```python
from build123d import *

# Parameters (mm, degrees)
SKETCH1_W           = 25.5
SKETCH1_H           = 5.5
BOSS_EXTRUDE1_DEPTH = 5


with BuildPart() as part:
    # Sketch1 → Boss-Extrude1 (new body)
    with BuildSketch(Plane.XY):
        Polygon((-100, 151.5), (-100, 146.5), (10, 146.5), (10, 151.5), (30, 151.5), (30, -10), (10, -10), (10, -5), (-100, -5), (-100, -10), (-120, -10), (-120, -5), (-115, -5), (-115, 146.5), (-120, 146.5), (-120, 151.5), align=None)
        with Locations((-58.25, 13.75)):
            Rectangle(SKETCH1_W, SKETCH1_H, mode=Mode.SUBTRACT)
        with Locations((-12.75, 2.75)):
            Rectangle(SKETCH1_W, SKETCH1_H, mode=Mode.SUBTRACT)
        with Locations((-58.25, 2.75)):
            Rectangle(SKETCH1_W, SKETCH1_H, mode=Mode.SUBTRACT)
        with Locations((-12.75, 13.75)):
            Rectangle(SKETCH1_W, SKETCH1_H, mode=Mode.SUBTRACT)
        with Locations((-12.75, 26.25)):
            Rectangle(SKETCH1_W, SKETCH1_H, mode=Mode.SUBTRACT)
        with Locations((-58.25, 26.25)):
            Rectangle(SKETCH1_W, SKETCH1_H, mode=Mode.SUBTRACT)
        with Locations((-58.25, 37.25)):
            Rectangle(SKETCH1_W, SKETCH1_H, mode=Mode.SUBTRACT)
        with Locations((-12.75, 37.25)):
            Rectangle(SKETCH1_W, SKETCH1_H, mode=Mode.SUBTRACT)
        with Locations((-12.75, 49.75)):
            Rectangle(SKETCH1_W, SKETCH1_H, mode=Mode.SUBTRACT)
        with Locations((-58.25, 49.75)):
            Rectangle(SKETCH1_W, SKETCH1_H, mode=Mode.SUBTRACT)
        with Locations((-58.25, 60.75)):
            Rectangle(SKETCH1_W, SKETCH1_H, mode=Mode.SUBTRACT)
        with Locations((-12.75, 60.75)):
            Rectangle(SKETCH1_W, SKETCH1_H, mode=Mode.SUBTRACT)
        with Locations((-12.75, 73.25)):
            Rectangle(SKETCH1_W, SKETCH1_H, mode=Mode.SUBTRACT)
        with Locations((-58.25, 73.25)):
            Rectangle(SKETCH1_W, SKETCH1_H, mode=Mode.SUBTRACT)
        with Locations((-58.25, 84.25)):
            Rectangle(SKETCH1_W, SKETCH1_H, mode=Mode.SUBTRACT)
        with Locations((-12.75, 84.25)):
            Rectangle(SKETCH1_W, SKETCH1_H, mode=Mode.SUBTRACT)
        with Locations((-12.75, 96.75)):
            Rectangle(SKETCH1_W, SKETCH1_H, mode=Mode.SUBTRACT)
        with Locations((-58.25, 96.75)):
            Rectangle(SKETCH1_W, SKETCH1_H, mode=Mode.SUBTRACT)
        with Locations((-58.25, 107.75)):
            Rectangle(SKETCH1_W, SKETCH1_H, mode=Mode.SUBTRACT)
        with Locations((-12.75, 107.75)):
            Rectangle(SKETCH1_W, SKETCH1_H, mode=Mode.SUBTRACT)
        with Locations((-12.75, 120.25)):
            Rectangle(SKETCH1_W, SKETCH1_H, mode=Mode.SUBTRACT)
        with Locations((-58.25, 120.25)):
            Rectangle(SKETCH1_W, SKETCH1_H, mode=Mode.SUBTRACT)
        with Locations((-58.25, 131.25)):
            Rectangle(SKETCH1_W, SKETCH1_H, mode=Mode.SUBTRACT)
        with Locations((-12.75, 131.25)):
            Rectangle(SKETCH1_W, SKETCH1_H, mode=Mode.SUBTRACT)
    extrude(amount=BOSS_EXTRUDE1_DEPTH)


solid = part.part
```
Build history of the part. All positions in model axes, mm. Coordinates: 2 decimals unless noted, no trailing zeros. Order: outer loops, then holes, each group sorted by start corner. A loop starts at its lowest first (then second) coordinate and runs counter-clockwise, first axis right, second up. Notation, with made-up numbers: (87.25, -2) -> (136.25, -2) arc R13 cw to (136.25, 23) -> close; hole circle Ø10 at (-38.75, 54). An arc over 180 degrees is marked (long way). Answer in a Markdown table with one row per item. Add a question column.
Q1. Band-saw the part on D-D, the plane x = -81. List the corners of the cut face in (y, z), then the cut area to 4 significant figures.
Q2. Mould opens along Y. For faces 1 (the face through (-45.5, 108, 2)), 2 (the face through (20, 151.5, 2)), 3 (the face through (10, -8, 2)) say: +Y half, -Y half, draft (parallel to the pull), parting line (faces both ways), or undercut.
Q3. Band-saw the part on A-A, the plane z = 1.7. Give the number of separate pieces and of enclosed holes in the cut face, then the cut area to 3 significant figures.
Q4. Drop flat-ended pins along their axis: pin 1 (2.5 mm diameter, centred on y = 119.5, z = 3, fed in from -X); pin 2 (2.5 mm diameter, centred on x = -6.5, z = 3, fed in from +Y). Give the stop position or say it passes through.
Q5. Wall check: line 1 along X through (y, z) = (95.5, 2.7); line 2 along X through (y, z) = (141, 4.1); line 3 along Y through (x, z) = (-73.5, 1.5). Give the ranges that are in metal, low to high. Write a range as [from, to].
Q6. Band-saw the part on C-C, the plane y = 115.5. List the corners of the cut face in (x, z), then the cut area to 3 significant figures.
Answers follow:
| question | item | result |
|---|---|---|
| 1 | outline | (-5, 0) -> (146.5, 0) -> (146.5, 5) -> (-5, 5) -> close |
| 1 | area | 757.5 mm^2 |
| 2 | face 1 | undercut |
| 2 | face 2 | +Y half |
| 2 | face 3 | draft |
| 3 | separate pieces | 1 |
| 3 | enclosed holes | 24 |
| 3 | area | 19,000 mm^2 |
| 4 | pin 1 | x = -115 |
| 4 | pin 2 | y = 146.5 |
| 5 | line 1 | [-115, -71], [-45.5, -25.5], [0, 30] |
| 5 | line 2 | [-115, 30] |
| 5 | line 3 | [-5, 146.5] |
| 6 | outline | (-115, 0) -> (30, 0) -> (30, 5) -> (-115, 5) -> close |
| 6 | area | 725 mm^2 |
